Input: dimensioned drawing with shaded views. Units: mm. Origin: part minimum x, y, z. A direction names the side the tool comes from. Coordinates: 2 decimals unless noted, no trailing zeros. Loops run counter-clockwise (first coordinate to the right, second up) from the corner with the lowest first, then second, coordinate; pieces in that order, holes last.
Item 1: Section query A-A, the plane x = 12. Return the cut outline in (y, z) (1 decimal).
Item 2: Section query C-C, the plane y = 28. Return the cut outline in (x, z).
Item 3: Section query D-D, the plane x = 20.5. Return the cut outline in (y, z) (1 decimal).
Item 4: Reachability of the marked faces 1, 2 and 3 from +Z, -Z, +X, -X, +Y, -Y: full face, straight path, thin tool, end or side. Return the list, or none.
Item 5: Pin query (flat end, axial travel): pin 1 Ø6 at (x, z) = (41, 12.5) entering from -Y; pin 2 Ø1 at (x, y) = (36, 8) entering from +Z; pin 3 Ø5 at (x, y) = (31.5, 8.5) entering from +Z. Return the tip coordinate at first contact, or that it passes through.
Item 6: Pull-direction query (X, two-part tool) for the marked faces 4, 5 and 6; classes: +X half, -X half, draft (parallel to the pull), parting line (faces both ways), or undercut.
Item 7: Section query B-B, the plane z = 4.5. Return the cut outline in (x, y).
Item 8: Line query: probe 1 along Z at (x, y) = (31, 36); probe 2 along Z at (x, y) = (34, 36) (1 decimal); probe 3 along X at (y, z) = (35.5, 6). Output: solid intervals per line, ascending.
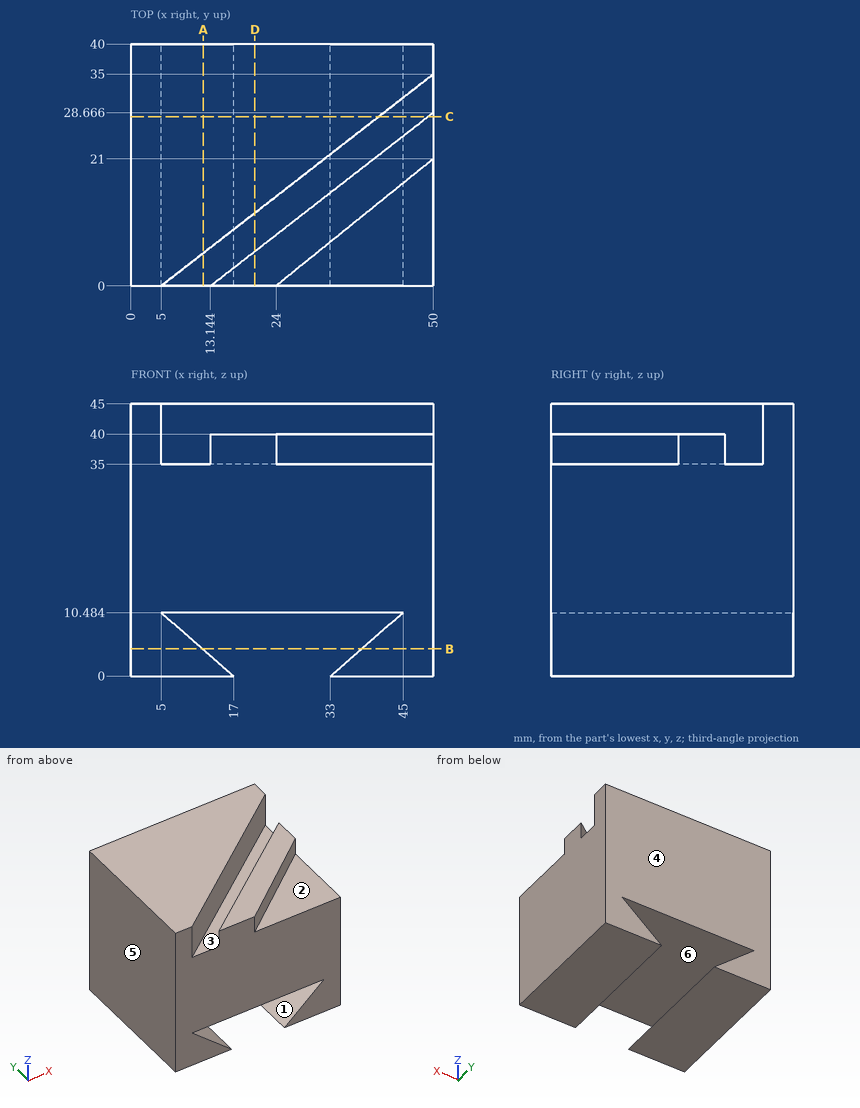
Verdict:
1. outline: (0, 0) - (40, 0) - (40, 4.4) - (0, 4.4) - close; (0, 10.5) - (40, 10.5) - (40, 45) - (5.4, 45) - (5.4, 35) - (0, 35) - close
2. outline: (0, 0) - (17, 0) - (5, 10.48) - (45, 10.48) - (33, 0) - (50, 0) - (50, 40) - (49.14, 40) - (49.14, 35) - (41, 35) - (41, 45) - (0, 45) - close
3. outline: (0, 10.5) - (40, 10.5) - (40, 45) - (12.1, 45) - (12.1, 35) - (5.7, 35) - (5.7, 40) - (0, 40) - close
4. face 1: +Y, -Y
4. face 2: +Z, +X, -Y
4. face 3: +Z
5. pin 1: stops at y = 0
5. pin 2: stops at z = 35
5. pin 3: stops at z = 40
6. face 4: draft
6. face 5: -X half
6. face 6: undercut
7. outline: (0, 0) - (11.85, 0) - (11.85, 40) - (0, 40) - close; (38.15, 0) - (50, 0) - (50, 40) - (38.15, 40) - close
8. probe 1: z = 10.48 to 45
8. probe 2: z = 0 to 0.9, 10.5 to 45
8. probe 3: x = 0 to 10.13, 39.87 to 50
